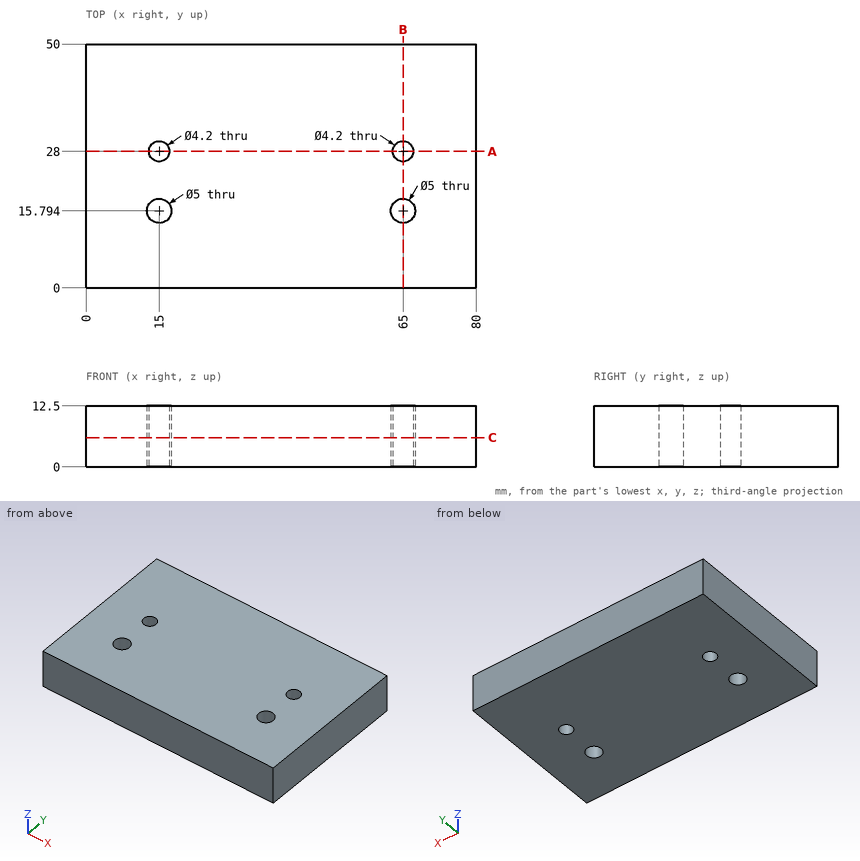
Design review of the part shown in the three views and the two pictorial views. Dimensions are in mm from the part's minimum x, y and z. Coordinates: 2 decimals unless noted, no trailing zeros. Order: outer loops, then holes, each group sorted by start corner. A loop starts at its lowest first (then second) coordinate and runs counter-clockwise, first axis right, second up.
Item 1: Take a section at B-B, the plane x = 65. Write out the cut boundary in (y, z), then the cut area to 3 significant figures.
Item 2: For line 1 (Y direction, x = 15, z = 7.5); line 2 (Y direction, x = 16, z = 6.75) (1 decimal), list the stretches that pass through material, from the lowest coordinate up.
Item 3: Take a section at C-C, the plane z = 6. Write out the cut boundary in (x, y).
Item 4: Take a section at A-A, the plane y = 28. Write out the cut boundary in (x, z).
The answers:
1. outline: (0, 0) - (13.29, 0) - (13.29, 12.5) - (0, 12.5) - close; (18.29, 0) - (25.9, 0) - (25.9, 12.5) - (18.29, 12.5) - close; (30.1, 0) - (50, 0) - (50, 12.5) - (30.1, 12.5) - close
1. area: 510 mm2
2. line 1: y = 0 to 13.29, 18.29 to 25.9, 30.1 to 50
2. line 2: y = 0 to 13.5, 18.1 to 26.2, 29.8 to 50
3. outline: (0, 0) - (80, 0) - (80, 50) - (0, 50) - close; hole circle Ø5 at (15, 15.79); hole circle Ø4.2 at (15, 28); hole circle Ø5 at (65, 15.79); hole circle Ø4.2 at (65, 28)
4. outline: (0, 0) - (12.9, 0) - (12.9, 12.5) - (0, 12.5) - close; (17.1, 0) - (62.9, 0) - (62.9, 12.5) - (17.1, 12.5) - close; (67.1, 0) - (80, 0) - (80, 12.5) - (67.1, 12.5) - close
